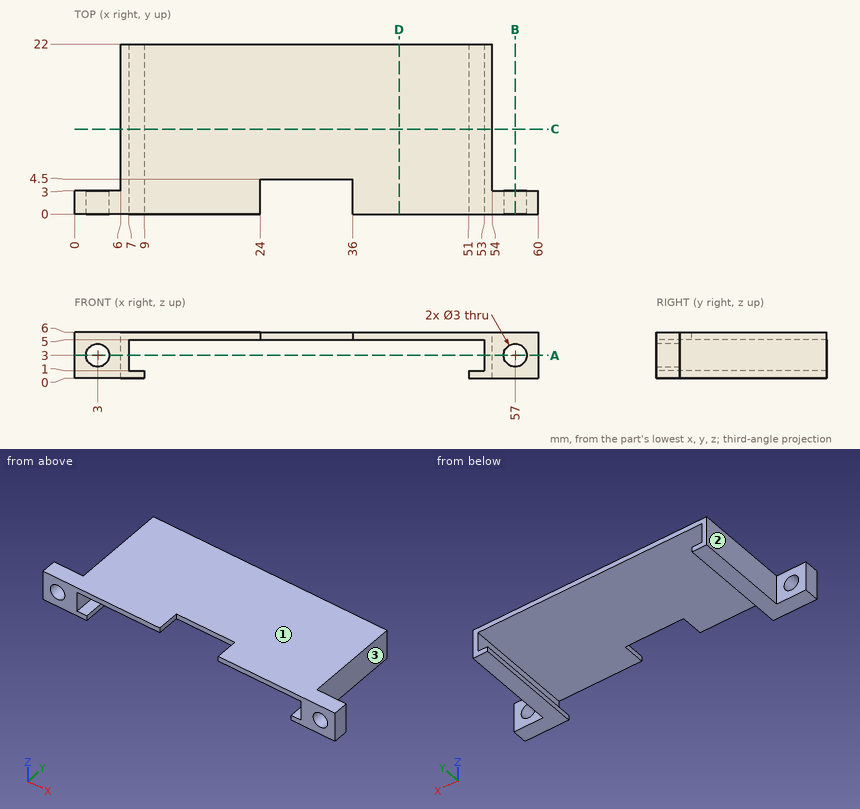
Source: three-view drawing plus pictorial views. Frame: mm from the lowest corner of the part. A direction names the side the tool comes from. Round coordinates to 2 decimals unless told otherwise and drop trailing zeros. Order: outer loops, then holes, each group sorted by start corner. A loop starts at its lowest first (then second) coordinate and runs counter-clockwise, first axis right, second up. Notation, with made-up numbers: (-1, 64) -> (23, 64) arc R20 ccw to (23, 97) -> close; hole circle Ø5 at (43, 75.25). An arc over 180 degrees is marked (long way). Use one line per item in the form item = value.
(1) Access query for the marked faces 1, 2 and 3. Directions: +Z, -Z, +X, -X, +Y, -Y. A direction counts if a zero-diameter tool reaches every point of the face in a straight line with its end or side. Return the directions, or none.
Results list:
face_1 = +Z, +X, -X, +Y, -Y
face_2 = +Z, -Z, -X, +Y
face_3 = +Z, -Z, +X, +Y
(2) Ray query, probe 1 along X at (y, z) = (18, 1.75); probe 2 along Z at (x, y) = (8, 19); probe 3 along Z at (x, y) = (21.5, 9.75). Return the intervals inside material, ascending. Write a range as [from, to].
Results list:
probe_1 = [6, 7], [53, 54]
probe_2 = [0, 1], [5, 6]
probe_3 = [5, 6]
(3) Section C-C on y = 11. Return loops of the section in (x, z), and give its area (3 significant figures).
Results list:
outline = (6, 0) -> (9, 0) -> (9, 1) -> (7, 1) -> (7, 5) -> (53, 5) -> (53, 1) -> (51, 1) -> (51, 0) -> (54, 0) -> (54, 6) -> (6, 6) -> close
area = 62.0 mm^2
(4) Section A-A on z = 3. Return loops of the section in (x, y).
Results list:
outline = (0, 0) -> (1.5, 0) -> (1.5, 3) -> (0, 3) -> close; (4.5, 0) -> (7, 0) -> (7, 22) -> (6, 22) -> (6, 3) -> (4.5, 3) -> close; (53, 0) -> (55.5, 0) -> (55.5, 3) -> (54, 3) -> (54, 22) -> (53, 22) -> close; (58.5, 0) -> (60, 0) -> (60, 3) -> (58.5, 3) -> close
(5) First-contact query: pin 1 Ø8 at (x, y) = (17.5, 13.5) entering from -Z; pin 2 Ø0.8 at (y, z) = (16, 0.5) entering from -X; pin 3 Ø0.8 at (y, z) = (3, 5.5) entering from -X; pin 4 Ø1.8 at (x, z) = (58, 1.5) entering from +Y. Flat tips, straight axial feed; report the tip coordinate or a pass-through.
Results list:
pin_1 = 5
pin_2 = 6
pin_3 = 0
pin_4 = 3
(6) Section D-D on x = 42. Return loops of the section in (y, z).
Results list:
outline = (0, 5) -> (22, 5) -> (22, 6) -> (0, 6) -> close
(7) Section B-B on x = 57. Return loops of the section in (y, z), and give its area (3 significant figures).
Results list:
outline = (0, 0) -> (3, 0) -> (3, 1.5) -> (0, 1.5) -> close; (0, 4.5) -> (3, 4.5) -> (3, 6) -> (0, 6) -> close
area = 9.00 mm^2
